from build123d import *

# Parameters (mm, degrees)
SKETCH_2_R      = 5
EXTRUDE_2_DEPTH = 5


with BuildPart() as part:
    # 草图1 → 旋转1 (revolve)
    with BuildSketch(Plane.XY):
        Polygon((0, 0), (0, 12), (19, 12), (19, 9), (33, 9), (33, 24), (35, 24), (35, 32.5), (223, 32.5), (223, 0), align=None)
    revolve(axis=Axis((223, 0, 0), (-1, 0, 0)))

    # 草图2 → 凸台-拉伸2 (add)
    with BuildSketch(Plane.ZY):
        with Locations(Location((0, 0, 0), (0, 0, 270))):
            Circle(SKETCH_2_R)
    extrude(amount=EXTRUDE_2_DEPTH)


solid = part.part
For this review, take the finished solid that the model builds, in its own axes (mm). A direction names the side the tool comes from. Give positions to 0.01 mm unless a question says otherwise; leave off trailing zeros. Loops run counter-clockwise (first coordinate to the right, second up) from the corner with the lowest first, then second, coordinate; pieces in that order, holes last.
Item 1: Take a section at A-A, the plane y = 0. State the section outline as (x, z) points.
Item 2: Take a section at D-D, the plane y = -14.5. State the section outline as (x, z) points.
Item 3: For line 1 along X through (y, z) = (-12, 23); line 2 along X through (y, z) = (-6, -8.5); line 3 along X through (y, z) = (13, -20), list the stretches that pass through material, from the lowest coordinate up.
Item 4: Take a section at C-C, the plane x = 45.5. State the section outline as (y, z) points, and give its area (3 significant figures).
Item 5: Insertion check: pin 1 (8 mm diameter, centred on x = 104.5, z = -8.5, fed in from +Y); pin 2 (1.5 mm diameter, centred on y = 4.5, z = -10.5, fed in from -X); pin 3 (4 mm diameter, centred on x = 109.5, z = 25, fed in from +Y). Each pin has a flat end and moves straight along its axis. Give the tip position at first contact, or say it passes through.
Item 6: Tool access review of faces 1 (the flat face through (35, 3, 24)), 2 (the flat face through (-5, 0, 0)), 3 (the flat face through (19, 2, -9)): name each direction out of +Z, -Z, +X, -X, +Y, -Y from which nothing blocks a thin tool from reaching the whole face with its end or side.
Calculated:
1. outline: (-5, -5) - (0, -5) - (0, -12) - (19, -12) - (19, -9) - (33, -9) - (33, -24) - (35, -24) - (35, -32.5) - (223, -32.5) - (223, 32.5) - (35, 32.5) - (35, 24) - (33, 24) - (33, 9) - (19, 9) - (19, 12) - (0, 12) - (0, 5) - (-5, 5) - close
2. outline: (33, -19.12) - (35, -19.12) - (35, -29.09) - (223, -29.09) - (223, 29.09) - (35, 29.09) - (35, 19.12) - (33, 19.12) - close
3. line 1: x = 35 to 223
3. line 2: x = 0 to 19, 33 to 223
3. line 3: x = 33 to 223
4. outline: circle Ø65 at (0, 0)
4. area: 3,320 mm2
5. pin 1: stops at y = 32.19
5. pin 2: stops at x = 0
5. pin 3: stops at y = 22.96
6. face 1: -X
6. face 2: +Z, -Z, -X, +Y, -Y
6. face 3: none
